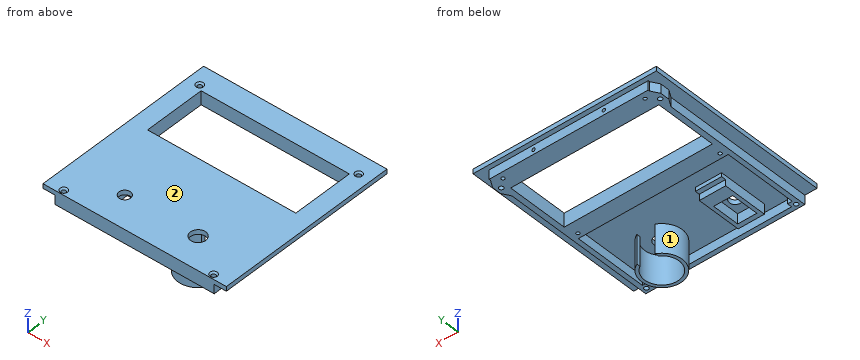
```python
from build123d import *

# Parameters (mm, degrees)
SZKIC1_W                        = 120
SZKIC1_H                        = 120
SZKIC1_R                        = 3.75
SZKIC1_R_2                      = 5
SZKIC1_W_2                      = 97
SZKIC1_H_2                      = 40
DODANIE_WYCI_GNI_CIE1_DEPTH     = 3
SZKIC1_4_W                      = 17.2
SZKIC1_4_H                      = 32
DODANIE_WYCI_GNI_CIE3_DEPTH     = 6.5
SZKIC1_7_W                      = 97
SZKIC1_7_H                      = 40
DODANIE_WYCI_GNI_CIE4_DEPTH     = 7
SZKIC9_W                        = 40
SZKIC9_H                        = 4
WYTNIJ_WYCI_GNI_CIE10_DEPTH     = 1
SZKIC7_R                        = 1.4
WYTNIJ_WYCI_GNI_CIE11_DEPTH     = 10
SZKIC1_8_R                      = 13.25
SZKIC1_8_R_2                    = 11.25
DODANIE_WYCI_GNI_CIE5_DEPTH     = 19
SZKIC11_W                       = 17.2
SZKIC11_H                       = 3
WYTNIJ_WYCI_GNI_CIE13_DEPTH     = 4
SZKIC12_W                       = 12
SZKIC12_H                       = 19
WYTNIJ_WYCI_GNI_CIE14_DEPTH     = 4
SZKIC13_R                       = 1.1
WYTNIJ_WYCI_GNI_CIE15_DEPTH     = 7
SZKIC14_W                       = 6
SZKIC14_H                       = 6
SZKIC14_R                       = 1.1
DODANIE_WYCI_GNI_CIE6_DEPTH     = 0.8
DODANIE_WYCI_GNI_CIE7_DEPTH     = 0.8
SFAZOWANIE1_SIZE                = 1
SFAZOWANIE2_SIZE                = 1
SFAZOWANIE3_SIZE                = 1
SFAZOWANIE4_SIZE                = 1
SZKIC17_R                       = 1.4
DODANIE_WYCI_GNI_CIE9_DEPTH     = 6
SZKIC18_W                       = 99.4
SZKIC18_H                       = 63.2
WYTNIJ_WYCI_GNI_CIE16_DEPTH     = 1
WYTNIJ_WYCI_GNI_CIE17_START     = -5
WYTNIJ_WYCI_GNI_CIE17_OUTLINE_R = 1.1
WYTNIJ_WYCI_GNI_CIE17_DEPTH     = 4.2


# Read off the part's stored shape, not the designer's step: Wytnij-wyci_gni_cie17
with BuildPart() as part:
    # Szkic1 → Dodanie-wyci_gni_cie1 (new body)
    with BuildSketch(Plane.XY):
        with Locations((60, 60)):
            Rectangle(SZKIC1_W, SZKIC1_H)
        with Locations((36, 20)):
            Circle(SZKIC1_R, mode=Mode.SUBTRACT)
        with Locations((84, 20)):
            Circle(SZKIC1_R_2, mode=Mode.SUBTRACT)
        with Locations((60, 85)):
            Rectangle(SZKIC1_W_2, SZKIC1_H_2, mode=Mode.SUBTRACT)
    extrude(amount=DODANIE_WYCI_GNI_CIE1_DEPTH)

    # Szkic1_7 → Dodanie-wyci_gni_cie4 (add)
    # profile 1 of 4: a face of its own
    with BuildSketch(Plane.XY):
        Polygon((11.5, 115), (10.3, 115), (10.3, 55), (11.5, 55), (108.5, 55), (109.7, 55), (109.7, 115), (108.5, 115), align=None)
        with Locations((60, 85)):
            Rectangle(SZKIC1_7_W, SZKIC1_7_H, mode=Mode.SUBTRACT)
    # profile 2 of 4: a face of its own
    with BuildSketch(Plane.XY):
        Polygon((11.5, 115), (10.3, 115), (10.3, 55), (11.5, 55), (108.5, 55), (109.7, 55), (109.7, 115), (108.5, 115), align=None)
        with Locations((60, 85)):
            Rectangle(SZKIC1_7_W, SZKIC1_7_H, mode=Mode.SUBTRACT)
    # profile 3 of 4: a face of its own
    with BuildSketch(Plane.XY):
        Polygon((11.5, 115), (10.3, 115), (10.3, 116.2), (109.7, 116.2), (109.7, 115), (108.5, 115), align=None)
    # profile 4 of 4: a face of its own
    with BuildSketch(Plane.XY):
        Polygon((10.3, 53.8), (109.7, 53.8), (109.7, 55), (108.5, 55), (11.5, 55), (10.3, 55), align=None)
    extrude(amount=-DODANIE_WYCI_GNI_CIE4_DEPTH)

    # Szkic9 → Wytnij-wyci_gni_cie10 (cut)
    with BuildSketch(Plane(origin=(0, 0, -7), x_dir=(-1, 0, 0), z_dir=(0, 0, -1))):
        with Locations((-40.5, 113)):
            Rectangle(SZKIC9_W, SZKIC9_H)
    extrude(amount=-WYTNIJ_WYCI_GNI_CIE10_DEPTH, mode=Mode.SUBTRACT)

    # Szkic7 → Wytnij-wyci_gni_cie11 (cut)
    with BuildSketch(Plane.XY.offset(3)):
        with Locations((11, 3)):
            Circle(SZKIC7_R)
        with Locations((109, 3)):
            Circle(SZKIC7_R)
        with Locations((8, 108)):
            Circle(SZKIC7_R)
        with Locations((112, 108)):
            Circle(SZKIC7_R)
    extrude(amount=-WYTNIJ_WYCI_GNI_CIE11_DEPTH, mode=Mode.SUBTRACT)

    # Szkic1_8 → Dodanie-wyci_gni_cie5 (add)
    with BuildSketch(Plane.XY):
        with Locations((84, 20)):
            Circle(SZKIC1_8_R)
        with Locations((84, 20)):
            Circle(SZKIC1_8_R_2, mode=Mode.SUBTRACT)
    extrude(amount=-DODANIE_WYCI_GNI_CIE5_DEPTH)

    # Szkic12 → Wytnij-wyci_gni_cie14 (cut)
    with BuildSketch(Plane(origin=(0, 33.25, 0), x_dir=(1, 0, 0), z_dir=(0, 1, 0))):
        with Locations((84, 9.5)):
            Rectangle(SZKIC12_W, SZKIC12_H)
    extrude(amount=-WYTNIJ_WYCI_GNI_CIE14_DEPTH, mode=Mode.SUBTRACT)

    # Szkic13 → Wytnij-wyci_gni_cie15 (cut)
    with BuildSketch(Plane(origin=(0, 0, -7), x_dir=(-1, 0, 0), z_dir=(0, 0, -1))):
        with Locations((-106.5, 113)):
            Circle(SZKIC13_R)
        with Locations((-13.5, 113)):
            Circle(SZKIC13_R)
        with Locations((-106.5, 57)):
            Circle(SZKIC13_R)
        with Locations((-13.5, 57)):
            Circle(SZKIC13_R)
    extrude(amount=-WYTNIJ_WYCI_GNI_CIE15_DEPTH, mode=Mode.SUBTRACT)

    # Szkic14 → Dodanie-wyci_gni_cie6 (add)
    # profile 1 of 2: a face of its own
    with BuildSketch(Plane(origin=(0, 116.2, 0), x_dir=(1, 0, 0), z_dir=(0, 1, 0))):
        with Locations((37, 3)):
            Rectangle(SZKIC14_W, SZKIC14_H)
        with Locations((37, 3)):
            Circle(SZKIC14_R, mode=Mode.SUBTRACT)
    # profile 2 of 2: a face of its own
    with BuildSketch(Plane(origin=(0, 116.2, 0), x_dir=(1, 0, 0), z_dir=(0, 1, 0))):
        with Locations((83, 3)):
            Rectangle(SZKIC14_W, SZKIC14_H)
        with Locations(Location((83, 3, 0), (0, 0, 180))):
            Circle(SZKIC14_R, mode=Mode.SUBTRACT)
    extrude(amount=DODANIE_WYCI_GNI_CIE6_DEPTH)

    # Szkic15 → Dodanie-wyci_gni_cie7 (add)
    with BuildSketch(Plane(origin=(0, 116.2, 0), x_dir=(1, 0, 0), z_dir=(0, 1, 0))):
        Polygon((109.7, 0), (109.7, 7), (10.3, 7), (10.3, 0), (34, 0), (34, 6), (40, 6), (40, 0), (80, 0), (80, 6), (86, 6), (86, 0), align=None)
    extrude(amount=DODANIE_WYCI_GNI_CIE7_DEPTH)

    # Sfazowanie1
    sfazowanie1_edges = [part.edges().sort_by_distance(p)[0] for p in [
        (6.6, 108, 3),
    ]]
    chamfer(sfazowanie1_edges, length=SFAZOWANIE1_SIZE)

    # Sfazowanie2
    sfazowanie2_edges = [part.edges().sort_by_distance(p)[0] for p in [
        (110.6, 108, 3),
    ]]
    chamfer(sfazowanie2_edges, length=SFAZOWANIE2_SIZE)

    # Sfazowanie3
    sfazowanie3_edges = [part.edges().sort_by_distance(p)[0] for p in [
        (9.6, 3, 3),
    ]]
    chamfer(sfazowanie3_edges, length=SFAZOWANIE3_SIZE)

    # Sfazowanie4
    sfazowanie4_edges = [part.edges().sort_by_distance(p)[0] for p in [
        (107.6, 3, 3),
    ]]
    chamfer(sfazowanie4_edges, length=SFAZOWANIE4_SIZE)


with BuildPart() as body_2:
    # Szkic1_4 → Dodanie-wyci_gni_cie3 (new body)
    with BuildSketch(Plane.XY):
        with Locations((36, 24)):
            Rectangle(SZKIC1_4_W, SZKIC1_4_H)
        Polygon((29.75, 11), (29.75, 26), (29.75, 29), (42.25, 29), (42.25, 26), (42.25, 11), align=None, mode=Mode.SUBTRACT)
    extrude(amount=-DODANIE_WYCI_GNI_CIE3_DEPTH)

    # Szkic11 → Wytnij-wyci_gni_cie13 (cut)
    with BuildSketch(Plane(origin=(0, 0, -6.5), x_dir=(-1, 0, 0), z_dir=(0, 0, -1))):
        with Locations((-36, 38.5)):
            Rectangle(SZKIC11_W, SZKIC11_H)
    extrude(amount=-WYTNIJ_WYCI_GNI_CIE13_DEPTH, mode=Mode.SUBTRACT)


    add(part.part)  # Dodanie-wyci_gni_cie9 merges part
    # Szkic17 → Dodanie-wyci_gni_cie9 (add)
    with BuildSketch(Plane(origin=(0, 0, 0), x_dir=(-1, 0, 0), z_dir=(0, 0, -1))):
        Polygon((-106.03246961, 3), (-106.03246961, 6), (-109.03246961, 6), (-109.03246961, 117), (-112.03246961, 117), (-112.03246961, 116.010548872), (-115.03246961, 111), (-115.03246961, 105), (-112.03246961, 99.989451128), (-112.03246961, 0), (-7.96753039, 0), (-7.96753039, 99.989451128), (-4.96753039, 105), (-4.96753039, 111), (-7.96753039, 116.010548872), (-7.96753039, 117), (-10.96753039, 117), (-10.96753039, 6), (-14.03246961, 6), (-14.03246961, 3), align=None)
        with Locations(Location((-112, 108, 0), (0, 0, 180))):
            Circle(SZKIC17_R, mode=Mode.SUBTRACT)
        with Locations(Location((-8, 108, 0), (0, 0, 180))):
            Circle(SZKIC17_R, mode=Mode.SUBTRACT)
        with Locations(Location((-11, 3, 0), (0, 0, 180))):
            Circle(SZKIC17_R, mode=Mode.SUBTRACT)
        with Locations(Location((-109, 3, 0), (0, 0, 180))):
            Circle(SZKIC17_R, mode=Mode.SUBTRACT)
    extrude(amount=DODANIE_WYCI_GNI_CIE9_DEPTH)

    # Szkic18 → Wytnij-wyci_gni_cie16 (cut)
    with BuildSketch(Plane(origin=(0, 0, -7), x_dir=(-1, 0, 0), z_dir=(0, 0, -1))):
        with Locations((-60, 85.4)):
            Rectangle(SZKIC18_W, SZKIC18_H)
    extrude(amount=-WYTNIJ_WYCI_GNI_CIE16_DEPTH, mode=Mode.SUBTRACT)

    # Wytnij-wyci_gni_cie17 outline → Wytnij-wyci_gni_cie17 (cut)
    with BuildSketch(Plane(origin=(0, 117, 0), x_dir=(1, 0, 0), z_dir=(0, 1, 0)).offset(WYTNIJ_WYCI_GNI_CIE17_START)):
        with Locations((37, 3)):
            Circle(WYTNIJ_WYCI_GNI_CIE17_OUTLINE_R)
        with Locations((83, 3)):
            Circle(WYTNIJ_WYCI_GNI_CIE17_OUTLINE_R)
    extrude(amount=WYTNIJ_WYCI_GNI_CIE17_DEPTH, mode=Mode.SUBTRACT)


solid = body_2.part
```
Here's how the part is built. I have some questions about the finished solid (model axes, mm). Face numbers are marked on the shaded views. Round coordinates to 2 decimals unless told otherwise and drop trailing zeros. Loops run counter-clockwise (first coordinate to the right, second up) from the corner with the lowest first, then second, coordinate; pieces in that order, holes last. Notation, with made-up numbers: (34, 80) -> (89, 80) arc R13 ccw to (89, 99) -> close; hole circle Ø10 at (-11.75, 69.25). An arc over 180 degrees is marked (long way). Answer as CSV lines item,"result". Start each with the question number.
1. Imagine slicing it at A-A on x = 101. Write out the boundary of the cut face in (y, z), plus the area to 3 significant figures.
2. Imagine slicing it at D-D on z = -12.5. Write out the boundary of the cut face in (x, y), plus the area to 3 significant figures.
3. I need wall thicknesses on probe 1 along Y at (x, z) = (11, -2.5); probe 2 along Y at (x, z) = (106.5, -3.2); probe 3 along Y at (x, z) = (25, -2). Which ranges of each line are inside material? Lowest first, please. Write a range as from..to.
4. I'm going to push flat-ended pins straight in: P1, Ø1.8, axis at y = 30.5, z = -13, coming from the +X side; P2, Ø1.5, axis at y = 26, z = -4.5, coming from the -X side; P3, Ø1.8, axis at x = 77.5, z = -2, coming from the +Y side. Where does each tip first touch, or does it pass through?
5. Imagine slicing it at C-C on y = 50.5. Write out the boundary of the cut face in (x, z), plus the area to 3 significant figures.
6. Imagine slicing it at B-B on y = 70. Write out the boundary of the cut face in (x, z).
7. If we mould it in two halves opening along Y, with no side actions, what happens to the marked faces 1 and 2? For each: pulls with the +Y half, pulls with the -Y half, needs draft (parallel to the pull), parting line crosses it, or undercut.
Solution:
1,outline,"(0, -6) -> (3, -6) -> (3, 0) -> (53.8, 0) -> (53.8, -6) -> (65, -6) -> (65, 3) -> (0, 3) -> close; (105, -6) -> (117, -6) -> (117, 0) -> (120, 0) -> (120, 3) -> (105, 3) -> close"
1,area,"397 mm²"
2,outline,"(78, 29.52) -> (78, 31.81) arc R13.25 ccw (long way) to (90, 31.81) -> (90, 29.52) arc R11.25 cw (long way) to start"
2,area,"129 mm²"
3,probe 1,"0..1.6, 4.4..6, 53.8..117"
3,probe 2,"0..6, 53.8..55.9, 58.1..65, 105..111.9, 114.1..117"
3,probe 3,"0..3, 53.8..65, 105..117"
4,P1,"x = 93.13"
4,P2,"x = 7.97"
4,P3,"y = 117"
5,outline,"(0, 0) -> (7.97, 0) -> (7.97, -6) -> (10.97, -6) -> (10.97, 0) -> (109.03, 0) -> (109.03, -6) -> (112.03, -6) -> (112.03, 0) -> (120, 0) -> (120, 3) -> (0, 3) -> close"
5,area,"396 mm²"
6,outline,"(0, 0) -> (7.97, 0) -> (7.97, -6) -> (11.5, -6) -> (11.5, 3) -> (0, 3) -> close; (108.5, -6) -> (112.03, -6) -> (112.03, 0) -> (120, 0) -> (120, 3) -> (108.5, 3) -> close"
7,face 1,"undercut"
7,face 2,"needs draft"
